Can you work these out from the model? Positions are in its coordinate system, mm. Give positions to 0.01 mm unless a question says otherwise; leave off trailing zeros. Loops run counter-clockwise (first coordinate to the right, second up) from the corner with the lowest first, then second, coordinate; pieces in that order, holes last.
from build123d import *

# Parameters (mm, degrees)
SKETCH_1_W      = 14.75
SKETCH_1_H      = 8
EXTRUDE_1_DEPTH = 1.2
SKETCH_2_W      = 14.75
SKETCH_2_H      = 3.9
EXTRUDE_2_DEPTH = 1.55
SKETCH_3_W      = 60
SKETCH_3_H      = 45
EXTRUDE_3_DEPTH = 1.3
FILLET_1_R      = 3
FILLET_2_R      = 1
FILLET_3_R      = 1


with BuildPart() as part:
    # 草图1 → 凸台-拉伸1 (new body)
    with BuildSketch(Plane(origin=(0, 0, 0), x_dir=(1, 0, 0), z_dir=(0, 1, 0))):
        Rectangle(SKETCH_1_W, SKETCH_1_H)
    extrude(amount=EXTRUDE_1_DEPTH)

    # 草图2 → 凸台-拉伸2 (add)
    with BuildSketch(Plane(origin=(0, 1.2, 0), x_dir=(1, 0, 0), z_dir=(0, 1, 0))):
        with Locations((0, 2.05)):
            Rectangle(SKETCH_2_W, SKETCH_2_H)
    extrude(amount=EXTRUDE_2_DEPTH)

    # 草图3 → 凸台-拉伸3 (add)
    with BuildSketch(Plane(origin=(0, 2.75, 0), x_dir=(1, 0, 0), z_dir=(0, 1, 0))):
        with Locations((0, -18.5)):
            Rectangle(SKETCH_3_W, SKETCH_3_H)
    extrude(amount=EXTRUDE_3_DEPTH)

    # 圆角1
    fillet_1_edges = [part.edges().sort_by_distance(p)[0] for p in [
        (0, 0, -4),
    ]]
    fillet(fillet_1_edges, radius=FILLET_1_R)

    # 圆角2
    fillet_2_edges = [part.edges().sort_by_distance(p)[0] for p in [
        (0, 1.2, 4),
    ]]
    fillet(fillet_2_edges, radius=FILLET_2_R)

    # 圆角3
    fillet_3_edges = [part.edges().sort_by_distance(p)[0] for p in [
        (0, 2.75, 41),
    ]]
    fillet(fillet_3_edges, radius=FILLET_3_R)


solid = part.part
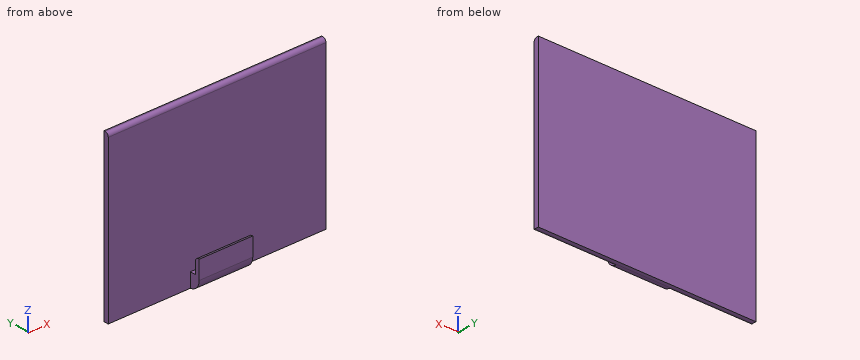
(1) Will these pins go through, and if not, where does the flat tip stop? P1, Ø6, axis at x = -14.5, z = 25, coming from the -Y side; P2, Ø1.2, axis at x = 3, y = 2, coming from the +Z side.
Returned:
P1: stops at y = 2.75
P2: stops at z = -0.1
(2) Please list where these lines run through material, in increasing order: probe 1 along Y at (x, z) = (10, 28.5); probe 2 along Z at (x, y) = (25.5, 3.7); probe 3 along Z at (x, y) = (-7, 2.65).
Returned:
probe 1: y = 2.75 to 4.05
probe 2: z = -4 to 41
probe 3: z = -3.98 to -0.1
(3) Suppose I cut it at B-B on z = 5. List the corners of the cut face in (x, y) for me, plus the area to 3 significant figures.
Returned:
outline: (-30, 2.75) - (30, 2.75) - (30, 4.05) - (-30, 4.05) - close
area: 78.0 mm2
(4) Suppose I cut it at A-A on x = 10.5. List the corners of the cut face in (y, z) for me, plus the area to 3 significant figures.
Returned:
outline: (2.75, -3.99) arc R3 ccw to (3, -4) - (4.05, -4) - (4.05, 41) - (3.75, 41) arc R1 ccw to (2.75, 40) - close
area: 58.3 mm2
(5) Suppose I cut it at C-C on x = 0.5. List the corners of the cut face in (y, z) for me, plus the area to 3 significant figures.
Returned:
outline: (0, -1) arc R3 ccw to (3, -4) - (4.05, -4) - (4.05, 41) - (3.75, 41) arc R1 ccw to (2.75, 40) - (2.75, -0.1) - (1.2, -0.1) - (1.2, 3) arc R1 ccw to (0.2, 4) - (0, 4) - close
area: 71.8 mm2
(6) Suppose I cut it at D-D on y = 2. List the corners of the cut face in (x, z) for me (3 decimals), plus the area to 3 significant figures.
Returned:
outline: (-7.375, -3.828) - (7.375, -3.828) - (7.375, -0.1) - (-7.375, -0.1) - close
area: 55.0 mm2
